Here's the drawing with two shaded views (mm, measured from the low corner). I have some questions. Give positions to 0.01 mm unless a question says otherwise; leave off trailing zeros. Write each loop counter-clockwise with the first axis right and the second up, starting at its lowest first coordinate (ties: lowest second). Pieces come first, ordered by that corner, then holes.
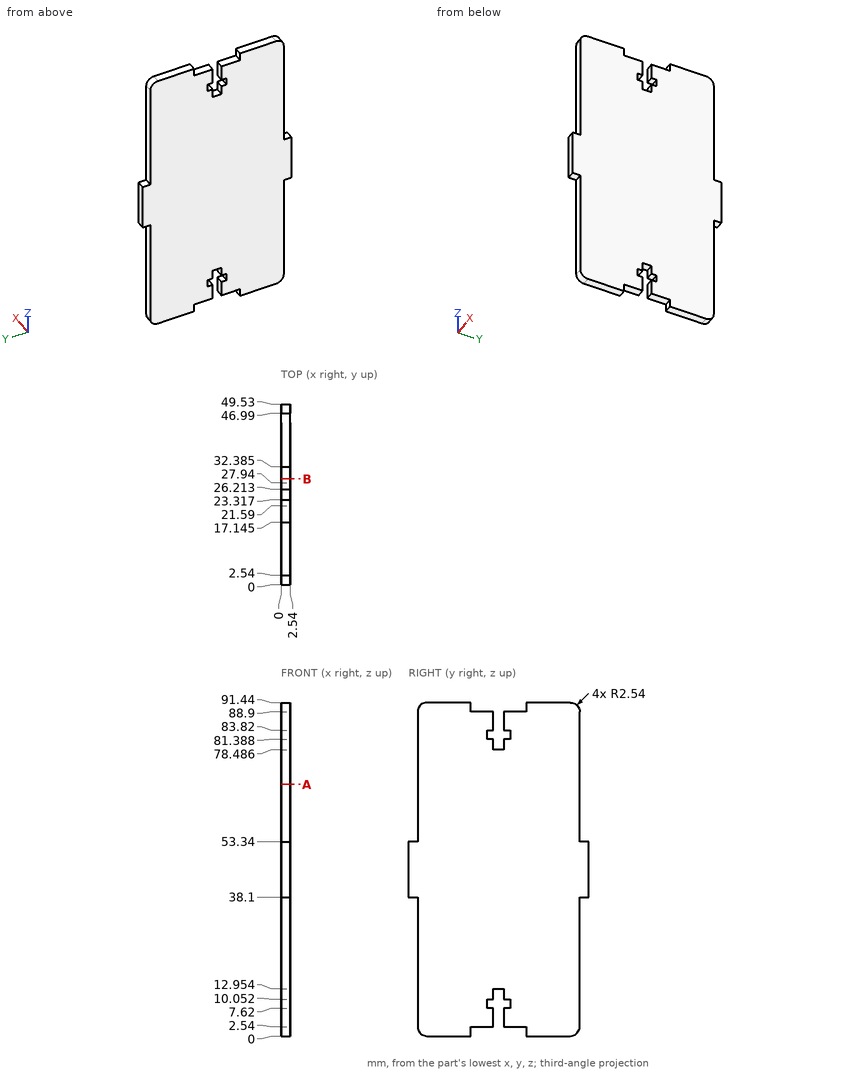
1) Suppose I cut it at A-A on z = 69. Write out the boundary of the cut face in (x, y).
Values follow:
outline: (0, 2.54) - (2.54, 2.54) - (2.54, 46.99) - (0, 46.99) - close
2) Please list where these lines run through material, in increasing order: L1, parallel to Y at x = 2.35, z = 8; L2, parallel to Y at x = 0.65, z = 12; L3, parallel to Y at x = 2.05, z = 78.
Values follow:
L1: y = 2.54 to 21.59, 27.94 to 46.99
L2: y = 2.54 to 23.32, 26.21 to 46.99
L3: y = 2.54 to 46.99
3) Suppose I cut it at B-B on y = 29. Write out the boundary of the cut face in (x, z).
Values follow:
outline: (0, 2.54) - (2.54, 2.54) - (2.54, 88.9) - (0, 88.9) - close
4) For pin 1 Ø1.3 at (x, y) = (1.5, 24.5) entering from -Z; pin 2 Ø0.8 at (x, z) = (2, 4.5) entering from +Y; pin 3 Ø1.4 at (x, y) = (1.5, 26.5) entering from +Z, each with a flat end and sliding along its axis, tell me the tip position at first contact or that it passes through.
Values follow:
pin 1: stops at z = 12.95
pin 2: stops at y = 46.99
pin 3: stops at z = 88.9
